Read the model definition and answer for the solid it produces. Units are mm, in the model's axes. Round coordinates to 2 decimals unless told otherwise and drop trailing zeros. Order: outer loops, then holes, each group sorted by start corner. A loop starts at its lowest first (then second) coordinate and runs counter-clockwise, first axis right, second up.
from build123d import *

# Parameters (mm, degrees)
F1_DEPTH = 2
F2_R     = 3
F3_DEPTH = 2
F4_R     = 1.525
F5_DEPTH = 2


with BuildPart() as f1:
    # F0 (on Top) → F1 (new body)
    with BuildSketch(Plane.XY):
        with BuildLine():
            Line((282, 0), (3, 0))
            ThreePointArc((3, 0), (0.87868, -0.87868), (0, -3))
            Line((0, -3), (0, -148))
            ThreePointArc((0, -148), (0.87868, -150.12132), (3, -151))
            Line((3, -151), (282, -151))
            ThreePointArc((282, -151), (284.12132, -150.12132), (285, -148))
            Line((285, -148), (285, -3))
            ThreePointArc((285, -3), (284.12132, -0.87868), (282, 0))
        make_face()
    extrude(amount=F1_DEPTH)

    # F2 (on face) → F3 (cut)
    with BuildSketch(Plane.XY.offset(2)):
        with Locations((8.5, -8.5)):
            Circle(F2_R)
        with Locations((8.5, -75.5)):
            Circle(F2_R)
        with Locations((8.5, -142.5)):
            Circle(F2_R)
        with Locations((276.5, -142.5)):
            Circle(F2_R)
        with Locations((276.5, -75.5)):
            Circle(F2_R)
        with Locations((276.5, -8.5)):
            Circle(F2_R)
    extrude(amount=-F3_DEPTH, mode=Mode.SUBTRACT)

    # F4 (on face) → F5 (cut)
    with BuildSketch(Plane.XY.offset(2)):
        with Locations((156, -63.1)):
            Circle(F4_R)
        with Locations((156, -25)):
            Circle(F4_R)
    extrude(amount=-F5_DEPTH, mode=Mode.SUBTRACT)


solid = f1.part
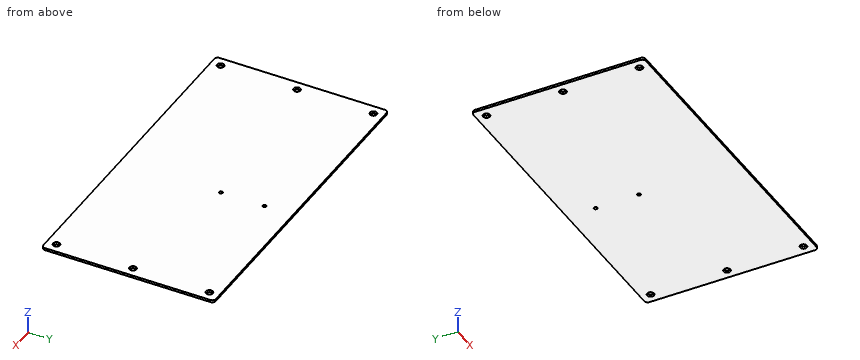
Q1. A cutting plane is placed at B-B, the plane x = 276.5. Give the vertices of the cut face in (y, z), plus the area to 3 significant figures.
Outcome:
outline: (-151, 0) - (-145.5, 0) - (-145.5, 2) - (-151, 2) - close; (-139.5, 0) - (-78.5, 0) - (-78.5, 2) - (-139.5, 2) - close; (-72.5, 0) - (-11.5, 0) - (-11.5, 2) - (-72.5, 2) - close; (-5.5, 0) - (0, 0) - (0, 2) - (-5.5, 2) - close
area: 266 mm2
Q2. A flat-ended cylindrical pin translates along its axis: pin 1 (2.5 mm diameter, centred on x = 156, y = -63.1, fed in from +Z). Find the tip coordinate at first contact, or state that the pin passes through.
Outcome:
pin 1: passes through
Q3. Straight lines are drawn through the part: probe 1 along X at (y, z) = (-142.5, 0.8); probe 2 along Y at (x, z) = (276.5, 0.95); probe 3 along X at (y, z) = (-63.5, 0.7). For each, find the intervals that lie inside material, in ascending order.
Outcome:
probe 1: x = 0 to 5.5, 11.5 to 273.5, 279.5 to 285
probe 2: y = -151 to -145.5, -139.5 to -78.5, -72.5 to -11.5, -5.5 to 0
probe 3: x = 0 to 154.53, 157.47 to 285
Q4. A cutting plane is placed at A-A, the plane y = -142.5. Give the vertices of the cut face in (x, z).
Outcome:
outline: (0, 0) - (5.5, 0) - (5.5, 2) - (0, 2) - close; (11.5, 0) - (273.5, 0) - (273.5, 2) - (11.5, 2) - close; (279.5, 0) - (285, 0) - (285, 2) - (279.5, 2) - close
